Answer from the drawing. Dimensions are ordinates in mm from the lowest x, y and z of the part. Round coordinates to 2 decimals unless told otherwise and drop trailing zeros. Loops run counter-clockwise (first coordinate to the right, second up) from the corner with the lowest first, then second, coordinate; pieces in that order, holes last. Notation, with made-up numbers: (1.25, 77.5) - (21.25, 77.5) arc R7 ccw to (21.25, 83.5) - close; hole circle Ø6 at (-30, 89). An arc over 180 degrees is marked (long way). Use CSV: the item, a comma, the result in double quotes. Start each with the question number.
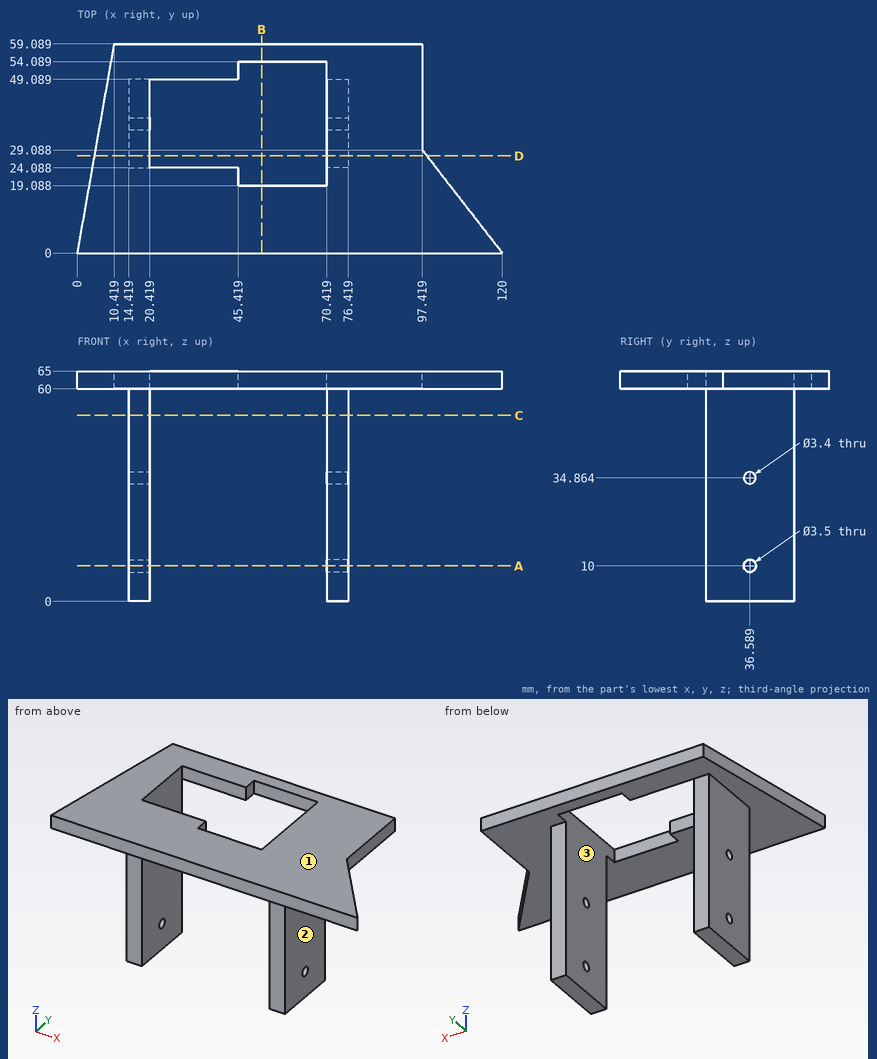
Item 1: Find the intervals of material crossed by probe 1 along X at (y, z) = (24.5, 43.5); probe 2 along Y at (x, z) = (24, 62.5); probe 3 along Y at (x, z) = (72, 10), in increasing order. Write a range as [from, to].
Item 2: A cutting plane is placed at A-A (z = 10). Determine the outline of the cut face in (x, y), plus the area to 3 significant figures.
Item 3: Each of these flat-tipped pins is pushed along its axis until it touches: pin 1 Ø12 at (x, y) = (25, 24) entering from -Z; pin 2 Ø1.8 at (x, z) = (17, 19) entering from -Y; pin 3 Ø2 at (x, y) = (66.5, 19) entering from -Z; pin 4 Ø12.5 at (y, z) = (35, 18) entering from +X. Where does it stop, or does it pass through?
Item 4: A cutting plane is placed at B-B (x = 52). Determine the outline of the cut face in (y, z).
Item 5: A cutting plane is placed at C-C (z = 52.5). Determine the outline of the cut face in (x, y), plus the area to 3 significant figures.
Item 6: A cutting plane is placed at D-D (y = 27.5). Determine the outline of the cut face in (x, z), plus the area to 3 significant figures.
Item 7: The mould has two halves that part along X. Classify the marked faces 1, 2 and 3: pulls with the +X half, pulls with the -X half, needs draft (parallel to the pull), parting line crosses it, or undercut.
Result sheet:
1,probe 1,"[14.42, 20.42], [70.42, 76.42]"
1,probe 2,"[0, 24.09], [49.09, 59.09]"
1,probe 3,"[24.09, 34.84], [38.34, 49.09]"
2,outline,"(14.42, 24.09) - (20.42, 24.09) - (20.42, 34.84) - (14.42, 34.84) - close; (14.42, 38.34) - (20.42, 38.34) - (20.42, 49.09) - (14.42, 49.09) - close; (70.42, 24.09) - (76.42, 24.09) - (76.42, 34.84) - (70.42, 34.84) - close; (70.42, 38.34) - (76.42, 38.34) - (76.42, 49.09) - (70.42, 49.09) - close"
2,area,"258 mm^2"
3,pin 1,"z = 0"
3,pin 2,"y = 24.09"
3,pin 3,"z = 60"
3,pin 4,"x = 76.42"
4,outline,"(0, 60) - (19.09, 60) - (19.09, 65) - (0, 65) - close; (54.09, 60) - (59.09, 60) - (59.09, 65) - (54.09, 65) - close"
5,outline,"(14.42, 24.09) - (20.42, 24.09) - (20.42, 49.09) - (14.42, 49.09) - close; (70.42, 24.09) - (76.42, 24.09) - (76.42, 49.09) - (70.42, 49.09) - close"
5,area,"300 mm^2"
6,outline,"(4.85, 60) - (14.42, 60) - (14.42, 0) - (20.42, 0) - (20.42, 65) - (4.85, 65) - close; (70.42, 0) - (76.42, 0) - (76.42, 60) - (98.65, 60) - (98.65, 65) - (70.42, 65) - close"
6,area,"939 mm^2"
7,face 1,"needs draft"
7,face 2,"pulls with the +X half"
7,face 3,"undercut"
